Check sheet for the modelled part. Datum: model origin and axes. Units: mm. A direction names the side the tool comes from. Round coordinates to 2 decimals unless told otherwise and drop trailing zeros. Write each loop counter-clockwise with the first axis right and the second up, starting at its lowest first coordinate (ties: lowest second). Pieces come first, ordered by that corner, then holes. Notation, with made-up numbers: M 25,80 L 68,80 A31 ccw 68,115 Z; hole C 67.25,69.25 d7. An arc over 180 degrees is marked long. One line per item, written item: value.
from build123d import *

# Parameters (mm, degrees)
F1_DEPTH = 25


with BuildPart() as f1:
    # F0 (on Front) → F1 (new body)
    with BuildSketch(Plane.XZ):
        with BuildLine():
            ThreePointArc((-5.038108, 28.560268), (-6.731504, 28.974006), (-8.464021, 28.78125))
            ThreePointArc((-8.464021, 28.78125), (-11.480503, 27.716386), (-14.366451, 26.336384))
            ThreePointArc((-14.366451, 26.336384), (-15.727824, 25.247608), (-16.632679, 23.757639))
            ThreePointArc((-16.632679, 23.757639), (-19.445436, 19.445436), (-23.757639, 16.632679))
            ThreePointArc((-23.757639, 16.632679), (-25.247608, 15.727824), (-26.336384, 14.366451))
            ThreePointArc((-26.336384, 14.366451), (-27.716386, 11.480503), (-28.78125, 8.464021))
            ThreePointArc((-28.78125, 8.464021), (-28.974006, 6.731504), (-28.560268, 5.038108))
            ThreePointArc((-28.560268, 5.038108), (-27.5, 0), (-28.560268, -5.038108))
            ThreePointArc((-28.560268, -5.038108), (-28.974006, -6.731504), (-28.78125, -8.464021))
            ThreePointArc((-28.78125, -8.464021), (-27.716386, -11.480503), (-26.336384, -14.366451))
            ThreePointArc((-26.336384, -14.366451), (-25.247608, -15.727824), (-23.757639, -16.632679))
            ThreePointArc((-23.757639, -16.632679), (-19.445436, -19.445436), (-16.632679, -23.757639))
            ThreePointArc((-16.632679, -23.757639), (-15.727824, -25.247608), (-14.366451, -26.336384))
            ThreePointArc((-14.366451, -26.336384), (-11.480503, -27.716386), (-8.464021, -28.78125))
            ThreePointArc((-8.464021, -28.78125), (-6.731504, -28.974006), (-5.038108, -28.560268))
            ThreePointArc((-5.038108, -28.560268), (0, -27.5), (5.038108, -28.560268))
            ThreePointArc((5.038108, -28.560268), (6.731504, -28.974006), (8.464021, -28.78125))
            ThreePointArc((8.464021, -28.78125), (11.480503, -27.716386), (14.366451, -26.336384))
            ThreePointArc((14.366451, -26.336384), (15.727824, -25.247608), (16.632679, -23.757639))
            ThreePointArc((16.632679, -23.757639), (19.445436, -19.445436), (23.757639, -16.632679))
            ThreePointArc((23.757639, -16.632679), (25.247608, -15.727824), (26.336384, -14.366451))
            ThreePointArc((26.336384, -14.366451), (27.716386, -11.480503), (28.78125, -8.464021))
            ThreePointArc((28.78125, -8.464021), (28.974006, -6.731504), (28.560268, -5.038108))
            ThreePointArc((28.560268, -5.038108), (27.5, 0), (28.560268, 5.038108))
            ThreePointArc((28.560268, 5.038108), (28.974006, 6.731504), (28.78125, 8.464021))
            ThreePointArc((28.78125, 8.464021), (27.716386, 11.480503), (26.336384, 14.366451))
            ThreePointArc((26.336384, 14.366451), (25.247608, 15.727824), (23.757639, 16.632679))
            ThreePointArc((23.757639, 16.632679), (19.445436, 19.445436), (16.632679, 23.757639))
            ThreePointArc((16.632679, 23.757639), (15.727824, 25.247608), (14.366451, 26.336384))
            ThreePointArc((14.366451, 26.336384), (11.480503, 27.716386), (8.464021, 28.78125))
            ThreePointArc((8.464021, 28.78125), (6.731504, 28.974006), (5.038108, 28.560268))
            ThreePointArc((5.038108, 28.560268), (0, 27.5), (-5.038108, 28.560268))
        make_face()
        Polygon((-20.06, -4.198434), (-20, -4.233075), (-17.56, -5.64181), (-17.56, -7), (-17.56, -8.528561), (-20.06, -9.971937), (-22.56, -8.528561), (-22.56, -5.64181), align=None, mode=Mode.SUBTRACT)
        Polygon((-8.06, -9.915313), (-10.56, -8.471937), (-10.56, -5.585186), (-8.06, -4.14181), (-5.56, -5.585186), (-5.56, -8.471937), align=None, mode=Mode.SUBTRACT)
        Polygon((6.44, -8.415313), (3.94, -9.858688), (1.44, -8.415313), (1.44, -5.528561), (3.94, -4.085186), (6.44, -5.528561), align=None, mode=Mode.SUBTRACT)
        Polygon((13.44, -8.358688), (13.44, -5.471937), (15.94, -4.028561), (18.44, -5.471937), (18.44, -8.358688), (15.94, -9.802064), align=None, mode=Mode.SUBTRACT)
        Polygon((-17.5, 6.443376), (-17.5, 3.556624), (-20, 2.113249), (-22.5, 3.556624), (-22.5, 6.443376), (-20, 7.886751), align=None, mode=Mode.SUBTRACT)
        Polygon((-10.5, 3.613249), (-10.5, 6.5), (-8, 7.943376), (-5.5, 6.5), (-5.5, 3.613249), (-8, 2.169873), align=None, mode=Mode.SUBTRACT)
        Polygon((1.5, 3.669873), (1.5, 6.556624), (4, 8), (6.5, 6.556624), (6.5, 3.669873), (4, 2.226497), align=None, mode=Mode.SUBTRACT)
        Polygon((13.5, 3.726497), (13.5, 6.613249), (16, 8.056624), (18.5, 6.613249), (18.5, 3.726497), (16, 2.283122), align=None, mode=Mode.SUBTRACT)
    extrude(amount=F1_DEPTH)


solid = f1.part
Q1. Scan lines: line 1 (X direction, y = -13.5, z = 5); line 2 (X direction, y = -7, z = -8); line 3 (Z direction, x = -21.5, y = -11.75). Record each from-to range of solid material in increasing order. Write a range as [from, to].
Completed:
line 1: [-28.54, -22.5], [-17.5, -10.5], [-5.5, 1.5], [6.5, 13.5], [18.5, 28.54]
line 2: [-28.89, -22.56], [-17.56, -10.56], [-5.56, 1.44], [6.44, 13.44], [18.44, 28.89]
line 3: [-17.79, -9.14], [-5.03, 2.98], [7.02, 17.79]
Q2. Draft check along X on faces 1 (the cylindrical face through (-25.27, -12.32, -15.71)), 2 (the flat face through (6.44, -12, -7)), 3 (the flat face through (1.44, -12, -7)), 4 (the cylindrical face through (15.744, -12.325, 25.229)). Enter one of: pulls with the +X half, pulls with the -X half, needs draft (parallel to the pull), parting line crosses it, or undercut.
Completed:
face 1: pulls with the -X half
face 2: undercut
face 3: undercut
face 4: pulls with the +X half
Q3. Access from +Z, -Z, +X, -X, +Y, -Y to the whole of each face (thin tool, end or side, straight path). Record for faces 5 (the cylindrical face through (-27.7, -12.32, 11.52)), 6 (the flat face through (-21.29, -12.32, -9.26)).
Completed:
face 5: +Z, -X, +Y, -Y
face 6: +Y, -Y
Q4. Sectioned sample at C-C on x = 0. Enter the section's corners in (y, z).
Completed:
outline: M -25,-27.5 L 0,-27.5 L 0,27.5 L -25,27.5 Z
Q5. Sectioned sample at B-B on x = -21.5. Enter the section's corners in (y, z), and give its area (3 significant figures).
Completed:
outline: M -25,-17.79 L 0,-17.79 L 0,-9.14 L -25,-9.14 Z; M -25,-5.03 L 0,-5.03 L 0,2.98 L -25,2.98 Z; M -25,7.02 L 0,7.02 L 0,17.79 L -25,17.79 Z
area: 685 mm^2
Q6. Sectioned sample at A-A on y = -7.75. State how many separate pieces and enclosed holes the cut face has, and give its area (3 significant figures).
Completed:
separate pieces: 1
enclosed holes: 8
area: 2,470 mm^2
Q7. Sectioned sample at D-D on z = -0.5. Enter the section's corners in (x, y), and give its area (3 significant figures).
Completed:
outline: M -27.51,-25 L 27.51,-25 L 27.51,0 L -27.51,0 Z
area: 1,380 mm^2
Q8. Depth check by flat-ended pin: P1, Ø3, axis at y = -13.5, z = 4.5, coming from the -X side; P2, Ø8, axis at y = -17, z = -23, coming from the -X side; P3, Ø6, axis at x = 12.5, y = -15, coming from the +Z side. Enter the tip coordinate at first touch or a pass-through.
Completed:
P1: x = -28.87
P2: x = -19.91
P3: z = 28.46
